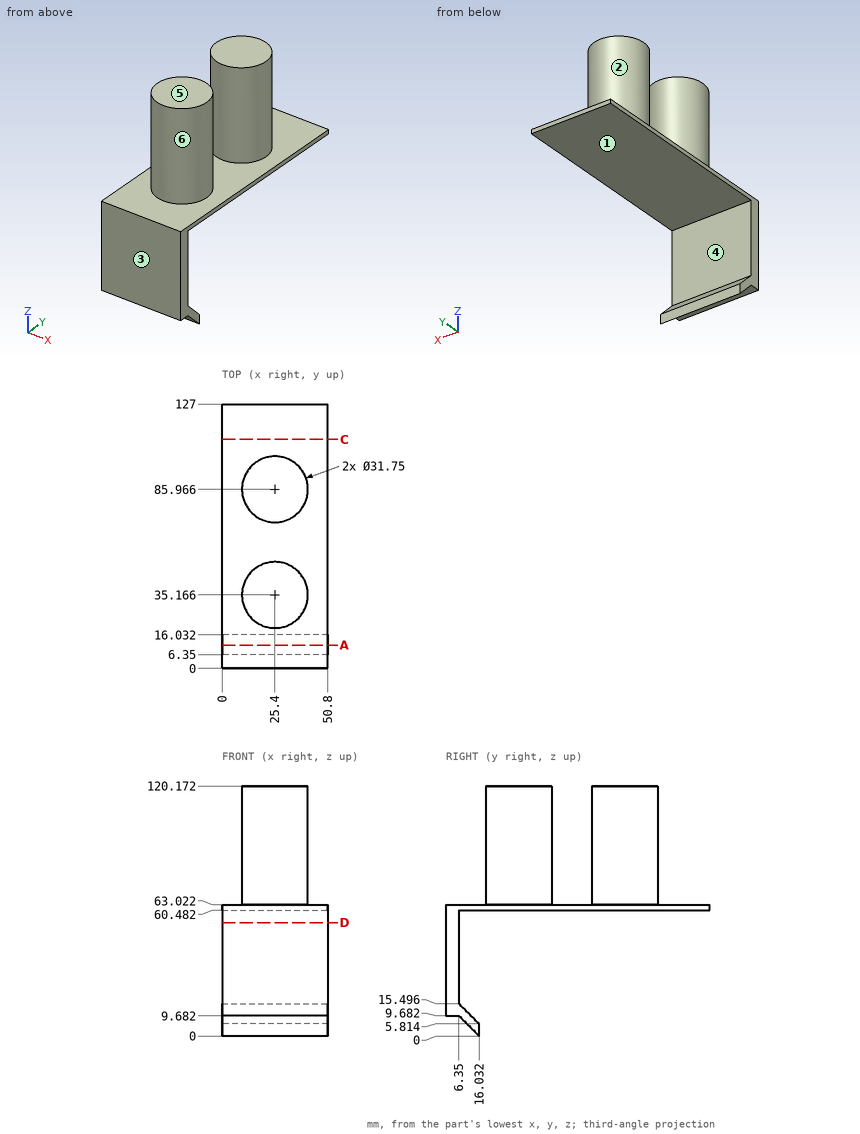
Geometry: see drawing. Coordinates: mm, zero at the bounding-box minimum. A direction names the side the tool comes from. Coordinates: 2 decimals unless noted, no trailing zeros. Loops run counter-clockwise (first coordinate to the right, second up) from the corner with the lowest first, then second, coordinate; pieces in that order, holes last. Notation, with made-up numbers: (35.5, 6) - (78.5, 6) arc R12 ccw to (78.5, 12) - close; hole circle Ø10 at (27, 59). An arc over 180 degrees is marked (long way). Put each result on its own line as item: value. Start each with the question number.
Q1. Line query: line 1 (Y direction, x = 34.5, z = 47); line 2 (Z direction, x = 7.5, y = 90); line 3 (Z direction, x = 10, y = 7) (1 decimal). Output: solid intervals per line, ascending.
Q2. Cut plane A-A, the plane y = 11. Return loops of the section in (x, z).
Q3. Cut plane C-C, the plane y = 110. Return loops of the section in (x, z), and give its area (3 significant figures).
Q4. Set-up query: the marked faces 4, 5 and 6. Return all of +Z, -Z, +X, -X, +Y, -Y with unobstructed straight access to the full face (end or side cutting, diameter ignored); none if empty.
Q5. Pin query (flat end, axial travel): pin 1 Ø5 at (x, y) = (30, 1.5) entering from -Z; pin 2 Ø6 at (x, z) = (34.5, 34.5) entering from +Y; pin 3 Ø6 at (x, y) = (15, 64) entering from -Z; pin 4 Ø1.5 at (x, z) = (12.5, 62.5) entering from -Y. Return the tip coordinate at first contact, or that it passes through.
Q6. Pull-direction query (Y, two-part tool) for the marked faces 1, 2 and 3; classes: released by +Y, released by -Y, zero draft, split by the parting line, or undercut.
Q7. Cut plane D-D, the plane z = 54.5. Return loops of the section in (x, y).
Filled sheet:
1. line 1: 0 to 6.35
1. line 2: 60.48 to 63.02
1. line 3: 9 to 14.8, 60.5 to 63
2. outline: (0, 5.03) - (50.8, 5.03) - (50.8, 10.85) - (0, 10.85) - close; (0, 60.48) - (50.8, 60.48) - (50.8, 63.02) - (0, 63.02) - close
3. outline: (0, 60.48) - (50.8, 60.48) - (50.8, 63.02) - (0, 63.02) - close
3. area: 129 mm²
4. face 4: +X, -X, +Y
4. face 5: +Z, +X, -X, +Y, -Y
4. face 6: +Z
5. pin 1: z = 9.68
5. pin 2: y = 6.35
5. pin 3: z = 60.48
5. pin 4: y = 0
6. face 1: zero draft
6. face 2: undercut
6. face 3: released by -Y
7. outline: (0, 0) - (50.8, 0) - (50.8, 6.35) - (0, 6.35) - close
